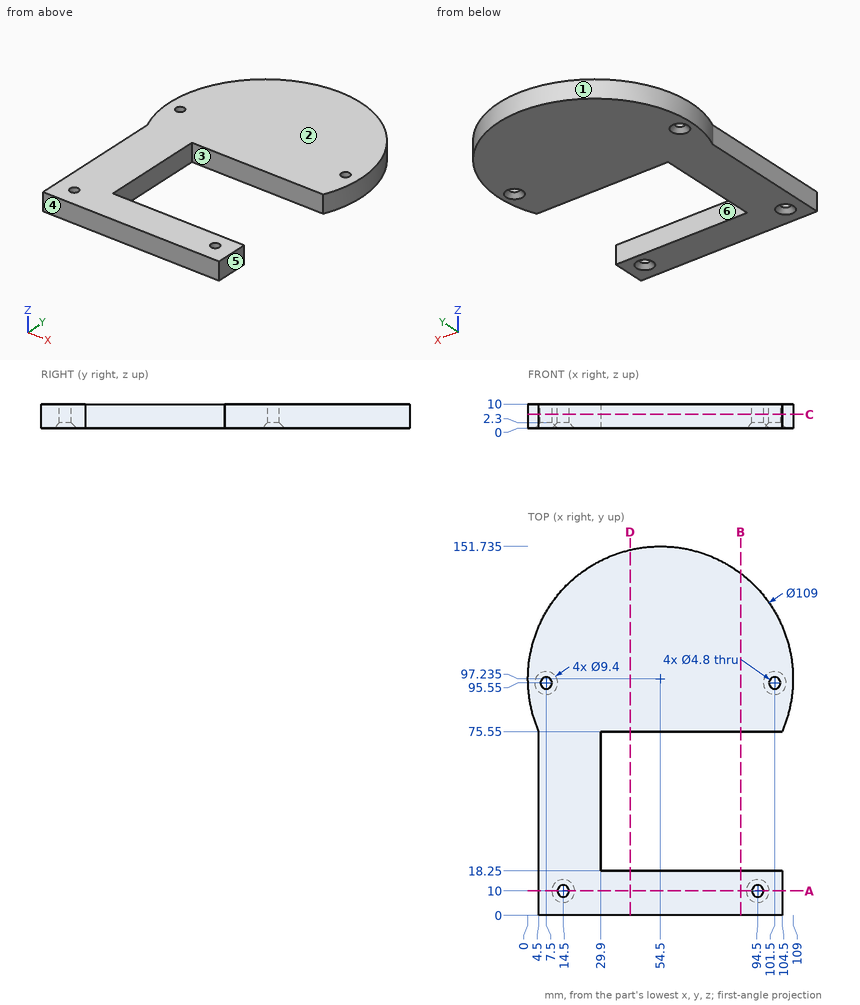
Print and shaded views of the part. All mm, measured from the part's lowest x, y and z. A direction names the side the tool comes from. Give positions to 0.01 mm unless a question says otherwise; leave off trailing zeros. Loops run counter-clockwise (first coordinate to the right, second up) from the corner with the lowest first, then second, coordinate; pieces in that order, holes last. Notation, with made-up numbers: (11, 80) -> (57, 80) arc R24 cw to (57, 95) -> close; hole circle Ø3 at (24, 13). An arc over 180 degrees is marked (long way). Answer in a Markdown table with one row per item.
Item 1: Slice it at A-A on y = 10. Write the cut outline in (x, z).
Findings below:
| item | result |
|---|---|
| outline | (4.5, 0) -> (9.8, 0) -> (12.1, 2.3) -> (12.1, 10) -> (4.5, 10) -> close; (16.9, 2.3) -> (19.2, 0) -> (89.8, 0) -> (92.1, 2.3) -> (92.1, 10) -> (16.9, 10) -> close; (96.9, 2.3) -> (99.2, 0) -> (104.5, 0) -> (104.5, 10) -> (96.9, 10) -> close |
Item 2: Slice it at C-C on z = 5.75. Give the number of separate pieces and of enclosed holes in the cut face, plus the area to 3 significant figures.
Findings below:
| item | result |
|---|---|
| separate pieces | 1 |
| enclosed holes | 4 |
| area | 10,200 mm² |
Item 3: Flat gauge pins, fed straight in: P1, Ø5, axis at x = 80, y = 91.5, coming from the -Z side; P2, Ø1, axis at y = 69.5, z = 1.5, coming from the +X side; P3, Ø3, axis at x = 85, z = 4, coming from the +Y side. Where does each tip first touch, or does it go through?
Findings below:
| item | result |
|---|---|
| P1 | stops at z = 0 |
| P2 | stops at x = 29.9 |
| P3 | stops at y = 143.38 |
Item 4: Mould opens along Y. For the marked faces 1, 2 and 3 say: pulls with the +Y half, pulls with the -Y half, needs draft (parallel to the pull), parting line crosses it, or undercut.
Findings below:
| item | result |
|---|---|
| face 1 | parting line crosses it |
| face 2 | needs draft |
| face 3 | undercut |
Item 5: Slice it at D-D on x = 42. Write the cut outline in (y, z), plus the area to 3 significant figures.
Findings below:
| item | result |
|---|---|
| outline | (0, 0) -> (18.25, 0) -> (18.25, 10) -> (0, 10) -> close; (75.55, 0) -> (150.28, 0) -> (150.28, 10) -> (75.55, 10) -> close |
| area | 930 mm² |
Item 6: Tool access for the marked faces 4, 5 and 6: list every direction of +Z, -Z, +X, -X, +Y, -Y with a clear straight run to the whole face (end or side of a thin tool).
Findings below:
| item | result |
|---|---|
| face 4 | +Z, -Z, +X, -X, -Y |
| face 5 | +Z, -Z, +X, -Y |
| face 6 | +Z, -Z, +X |
Item 7: Probe line 1 along X through (y, z) = (10, 7); line 2 along X through (y, z) = (70.5, 1.5); line 3 along Y through (x, z) = (62, 6.75). List the from-to ranges inside material, lowest first. Write a range as [from, to].
Findings below:
| item | result |
|---|---|
| line 1 | x = [4.5, 12.1], [16.9, 92.1], [96.9, 104.5] |
| line 2 | x = [4.5, 29.9] |
| line 3 | y = [0, 18.25], [75.55, 151.22] |
Item 8: Slice it at B-B on x = 87.5. Write the cut outline in (y, z), plus the area to 3 significant figures.
Findings below:
| item | result |
|---|---|
| outline | (0, 0) -> (18.25, 0) -> (18.25, 10) -> (0, 10) -> close; (75.55, 0) -> (140.61, 0) -> (140.61, 10) -> (75.55, 10) -> close |
| area | 833 mm² |
